Read the model definition and answer for the solid it produces. Units are mm, in the model's axes. Face numbers are marked on the shaded views. Round coordinates to 2 decimals unless told otherwise and drop trailing zeros. Order: outer loops, then holes, each group sorted by start corner. A loop starts at its lowest first (then second) coordinate and runs counter-clockwise, first axis right, second up. Notation, with made-up numbers: (-5, -24.5) - (39, -24.5) arc R28 cw to (39, -6.5) - close; hole circle Ø9 at (-37, -35). An arc over 180 degrees is marked (long way). Put each result on its own line as item: value. Start each with the question number.
Q1. Find the intervals of material crossed by line 1 along Z through (x, y) = (0.5, 52); line 2 along Z through (x, y) = (1, 12); line 3 along X through (y, z) = (-11, 0), in increasing order. Write a range as from..to.
Q2. Section A-A on y = 52 is taken. Give the vertices of the cut face in (x, z) (3 decimals).
Q3. Section D-D on x = 18.5 is taken. Give the vertices of the cut face in (y, z), then the cut area to 3 significant figures.
Q4. Section B-B on x = 0 is taken. Give the vertices of the cut face in (y, z), then the cut area to 3 significant figures.
Q5. Each of these flat-tipped pins is pushed along its axis until it touches: pin 1 Ø1.2 at (y, z) = (55.5, 7.5) entering from +X; pin 2 Ø10 at (x, z) = (17, 30.5) entering from +Y; pin 3 Ø4 at (y, z) = (11.5, 9) entering from -X. Where does it stop, or does it pass through?
Q6. For a pull along Y with two mould halves and no side action, classify the marked faces 1, 2 and 3 as pulls with the +Y half, pulls with the -Y half, needs draft (parallel to the pull), parting line crosses it, or undercut.
Q7. Section C-C on y = -8.5 is taken. State how many separate pieces and enclosed holes the cut face has, then the cut area to 3 significant figures.
from build123d import *

# Parameters (mm, degrees)
SKETCH1_R           = 25.3
BOSS_EXTRUDE1_DEPTH = 8.5
SKETCH2_R           = 25.3
BOSS_EXTRUDE2_DEPTH = 57.15
SKETCH7_R           = 25.3
BOSS_EXTRUDE4_DEPTH = 15
CUT_EXTRUDE3_DEPTH  = 115
SKETCH6_R           = 38.1
BOSS_EXTRUDE3_DEPTH = 15
CUT_EXTRUDE4_DEPTH  = 20
SKETCH10_R          = 2.75
CUT_EXTRUDE6_DEPTH  = 129
BOSS_EXTRUDE5_START = -93
BOSS_EXTRUDE5_DEPTH = 93
CUT_EXTRUDE7_DEPTH  = 40
CUT_EXTRUDE8_START  = -10
SKETCH12_R          = 25.3
CUT_EXTRUDE8_DEPTH  = 10


with BuildPart() as part:
    # Sketch1 → Boss-Extrude1 (new body)
    with BuildSketch(Plane(origin=(0, 0, 0), x_dir=(1, 0, 0), z_dir=(0, 1, 0))):
        with Locations(Location((0, 0, 0), (0, 0, 270))):
            Circle(SKETCH1_R)
    extrude(amount=BOSS_EXTRUDE1_DEPTH)

    # Sketch2 → Boss-Extrude2 (add)
    with BuildSketch(Plane(origin=(0, 8.5, 0), x_dir=(1, 0, 0), z_dir=(0, 1, 0))):
        with Locations(Location((0, 0, 0), (0, 0, 270))):
            Circle(SKETCH2_R)
    extrude(amount=BOSS_EXTRUDE2_DEPTH)

    # Sketch7 → Boss-Extrude4 (add)
    with BuildSketch(Plane(origin=(0, 65.65, 0), x_dir=(1, 0, 0), z_dir=(0, 1, 0))):
        with Locations(Location((0, 0, 0), (0, 0, 270))):
            Circle(SKETCH7_R)
    extrude(amount=BOSS_EXTRUDE4_DEPTH)

    # Sketch5 → Cut-Extrude3 (cut)
    with BuildSketch(Plane.XZ):
        with BuildLine():
            ThreePointArc((2.575, 6.777305881), (0, 7.25), (-2.575, 6.777305881))
            Line((-2.575, 6.777305881), (-2.575, 4))
            Line((-2.575, 4), (2.575, 4))
            Line((2.575, 4), (2.575, 6.777305881))
        make_face()
        with BuildLine():
            Line((-2.575, 4), (-2.575, 6.777305881))
            ThreePointArc((-2.575, 6.777305881), (-4.116658232, -5.96788279), (7.25, 0))
            ThreePointArc((7.25, 0), (5.96788279, 4.116658232), (2.575, 6.777305881))
            Line((2.575, 6.777305881), (2.575, 4))
            Line((2.575, 4), (-2.575, 4))
        make_face()
        with BuildLine():
            Line((2.575, 9.15), (-2.575, 9.15))
            Line((-2.575, 9.15), (-2.575, 6.777305881))
            ThreePointArc((-2.575, 6.777305881), (0, 7.25), (2.575, 6.777305881))
            Line((2.575, 6.777305881), (2.575, 9.15))
        make_face()
    extrude(amount=-CUT_EXTRUDE3_DEPTH, mode=Mode.SUBTRACT)

    # Sketch6 → Boss-Extrude3 (add)
    with BuildSketch(Plane.XZ):
        with Locations(Location((0, 0, 0), (0, 0, 270))):
            Circle(SKETCH6_R)
    extrude(amount=BOSS_EXTRUDE3_DEPTH)

    # Sketch9 → Cut-Extrude4 (cut)
    with BuildSketch(Plane(origin=(0, 0, 0), x_dir=(1, 0, 0), z_dir=(0, 1, 0))):
        with BuildLine():
            ThreePointArc((-23.75, 15.588457268), (-23.860741065, 16.429619165), (-24.185417438, 17.213457268))
            Line((-24.185417438, 17.213457268), (-27, 15.588457268))
            Line((-27, 15.588457268), (-27, 12.338457268))
            ThreePointArc((-27, 12.338457268), (-24.701902961, 13.290360229), (-23.75, 15.588457268))
        make_face()
        with BuildLine():
            Line((-27, 15.588457268), (-24.185417438, 17.213457268))
            ThreePointArc((-24.185417438, 17.213457268), (-29.814582562, 17.213457268), (-27, 12.338457268))
            Line((-27, 12.338457268), (-27, 15.588457268))
        make_face()
        with BuildLine():
            Line((2.814582562, 29.551914536), (0, 31.176914536))
            Line((0, 31.176914536), (-2.814582562, 29.551914536))
            ThreePointArc((-2.814582562, 29.551914536), (0, 27.926914536), (2.814582562, 29.551914536))
        make_face()
        with BuildLine():
            Line((-2.814582562, 29.551914536), (0, 31.176914536))
            Line((0, 31.176914536), (2.814582562, 29.551914536))
            ThreePointArc((2.814582562, 29.551914536), (3.139258935, 30.33575264), (3.25, 31.176914536))
            ThreePointArc((3.25, 31.176914536), (-0.841161897, 34.316173472), (-2.814582562, 29.551914536))
        make_face()
        with BuildLine():
            ThreePointArc((30.25, 15.588457268), (27.841161897, 18.727716204), (24.185417438, 17.213457268))
            Line((24.185417438, 17.213457268), (27, 15.588457268))
            Line((27, 15.588457268), (27, 12.338457268))
            ThreePointArc((27, 12.338457268), (29.298097039, 13.290360229), (30.25, 15.588457268))
        make_face()
        with BuildLine():
            Line((27, 15.588457268), (24.185417438, 17.213457268))
            ThreePointArc((24.185417438, 17.213457268), (24.185417438, 13.963457268), (27, 12.338457268))
            Line((27, 12.338457268), (27, 15.588457268))
        make_face()
        with BuildLine():
            ThreePointArc((30.25, -15.588457268), (29.298097039, -13.290360229), (27, -12.338457268))
            Line((27, -12.338457268), (27, -15.588457268))
            Line((27, -15.588457268), (24.185417438, -17.213457268))
            ThreePointArc((24.185417438, -17.213457268), (27.841161897, -18.727716204), (30.25, -15.588457268))
        make_face()
        with BuildLine():
            Line((27, -15.588457268), (27, -12.338457268))
            ThreePointArc((27, -12.338457268), (24.185417438, -13.963457268), (24.185417438, -17.213457268))
            Line((24.185417438, -17.213457268), (27, -15.588457268))
        make_face()
        with BuildLine():
            ThreePointArc((2.814582562, -29.551914536), (0, -27.926914536), (-2.814582562, -29.551914536))
            Line((-2.814582562, -29.551914536), (0, -31.176914536))
            Line((0, -31.176914536), (2.814582562, -29.551914536))
        make_face()
        with BuildLine():
            Line((0, -31.176914536), (-2.814582562, -29.551914536))
            ThreePointArc((-2.814582562, -29.551914536), (-0.841161897, -34.316173472), (3.25, -31.176914536))
            ThreePointArc((3.25, -31.176914536), (3.139258935, -30.33575264), (2.814582562, -29.551914536))
            Line((2.814582562, -29.551914536), (0, -31.176914536))
        make_face()
        with BuildLine():
            ThreePointArc((-23.75, -15.588457268), (-24.701902961, -13.290360229), (-27, -12.338457268))
            Line((-27, -12.338457268), (-27, -15.588457268))
            Line((-27, -15.588457268), (-24.185417438, -17.213457268))
            ThreePointArc((-24.185417438, -17.213457268), (-23.860741065, -16.429619165), (-23.75, -15.588457268))
        make_face()
        with BuildLine():
            Line((-27, -15.588457268), (-27, -12.338457268))
            ThreePointArc((-27, -12.338457268), (-29.814582562, -17.213457268), (-24.185417438, -17.213457268))
            Line((-24.185417438, -17.213457268), (-27, -15.588457268))
        make_face()
    extrude(amount=-CUT_EXTRUDE4_DEPTH, mode=Mode.SUBTRACT)

    # Sketch10 → Cut-Extrude6 (cut)
    with BuildSketch(Plane(origin=(0, 80.65, 0), x_dir=(1, 0, 0), z_dir=(0, 1, 0))):
        with Locations(Location((0, 15, 0), (0, 0, 270))):
            Circle(SKETCH10_R)
        with Locations(Location((0, -15, 0), (0, 0, 270))):
            Circle(SKETCH10_R)
    extrude(amount=-CUT_EXTRUDE6_DEPTH, mode=Mode.SUBTRACT)

    # Sketch11 → Boss-Extrude5 (add)
    with BuildSketch(Plane(origin=(0, 80.65, 0), x_dir=(1, 0, 0), z_dir=(0, 1, 0)).offset(BOSS_EXTRUDE5_START)):
        with BuildLine():
            ThreePointArc((7.25, 0), (-4.116658232, 5.96788279), (-2.575, -6.777305881))
            ThreePointArc((-2.575, -6.777305881), (0, -7.25), (2.575, -6.777305881))
            ThreePointArc((2.575, -6.777305881), (5.96788279, -4.116658232), (7.25, 0))
        make_face()
        with BuildLine():
            ThreePointArc((2.575, -6.777305881), (0, -7.25), (-2.575, -6.777305881))
            Line((-2.575, -6.777305881), (-2.575, -9.15))
            Line((-2.575, -9.15), (2.575, -9.15))
            Line((2.575, -9.15), (2.575, -6.777305881))
        make_face()
    extrude(amount=BOSS_EXTRUDE5_DEPTH)

    # Sketch11_3 → Cut-Extrude7 (cut)
    with BuildSketch(Plane(origin=(0, 80.65, 0), x_dir=(1, 0, 0), z_dir=(0, 1, 0))):
        with BuildLine():
            ThreePointArc((7.25, 0), (-4.116658232, 5.96788279), (-2.575, -6.777305881))
            ThreePointArc((-2.575, -6.777305881), (0, -7.25), (2.575, -6.777305881))
            ThreePointArc((2.575, -6.777305881), (5.96788279, -4.116658232), (7.25, 0))
        make_face()
        with BuildLine():
            ThreePointArc((2.575, -6.777305881), (0, -7.25), (-2.575, -6.777305881))
            Line((-2.575, -6.777305881), (-2.575, -9.15))
            Line((-2.575, -9.15), (2.575, -9.15))
            Line((2.575, -9.15), (2.575, -6.777305881))
        make_face()
    extrude(amount=-CUT_EXTRUDE7_DEPTH, mode=Mode.SUBTRACT)

    # Sketch12 → Cut-Extrude8 (cut)
    with BuildSketch(Plane(origin=(0, 80.65, 0), x_dir=(1, 0, 0), z_dir=(0, 1, 0)).offset(CUT_EXTRUDE8_START)):
        with Locations(Location((0, 0, 0), (0, 0, 270))):
            Circle(SKETCH12_R)
    extrude(amount=CUT_EXTRUDE8_DEPTH, mode=Mode.SUBTRACT)


solid = part.part
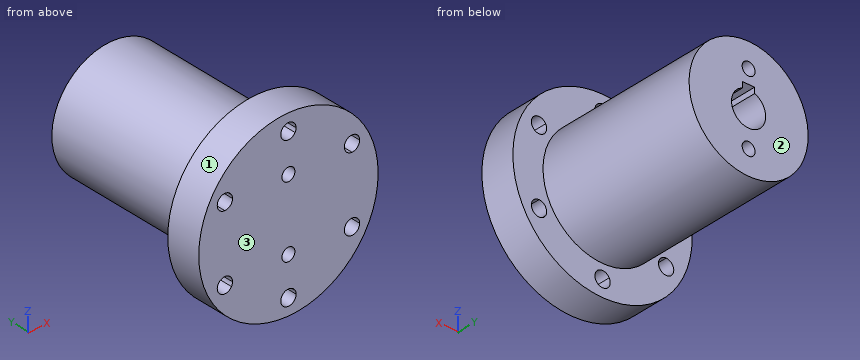
Findings:
1. line 1: -25.3..-17.7, -12.3..-7.23, 9.15..12.3, 17.7..25.3
1. line 2: -25.28..-17.56, -12.44..12.44, 17.56..25.28
1. line 3: -38.1..38.1
2. outline: circle Ø50.6 at (0, 0); hole circle Ø5.5 at (0, -15); hole circle Ø5.5 at (0, 15); hole (-2.575, 6.777) arc R7.25 ccw (long way) to (2.575, 6.777) - (2.575, 9.15) - (-2.575, 9.15) - close
3. outline: (-15, -33.31) - (0, -33.31) - (0, -17.26) - (70.65, -17.26) - (70.65, 17.26) - (0, 17.26) - (0, 33.31) - (-15, 33.31) - close
3. area: 3,440 mm2
4. outline: (-15, -38.1) - (0, -38.1) - (0, -34.43) - (-15, -34.43) - close; (-15, -27.93) - (0, -27.93) - (0, -25.3) - (70.65, -25.3) - (70.65, -17.75) - (-15, -17.75) - close; (-15, -12.25) - (70.65, -12.25) - (70.65, -7.25) - (40.65, -7.25) - (40.65, 9.15) - (70.65, 9.15) - (70.65, 12.25) - (-15, 12.25) - close; (-15, 17.75) - (70.65, 17.75) - (70.65, 25.3) - (0, 25.3) - (0, 27.93) - (-15, 27.93) - close; (-15, 34.43) - (0, 34.43) - (0, 38.1) - (-15, 38.1) - close
4. area: 3,090 mm2
5. pin 1: x = 24.34
5. pin 2: y = 0
5. pin 3: x = -24.31
6. face 1: needs draft
6. face 2: pulls with the +Y half
6. face 3: pulls with the -Y half
7. separate pieces: 1
7. enclosed holes: 8
7. area: 4,310 mm2
